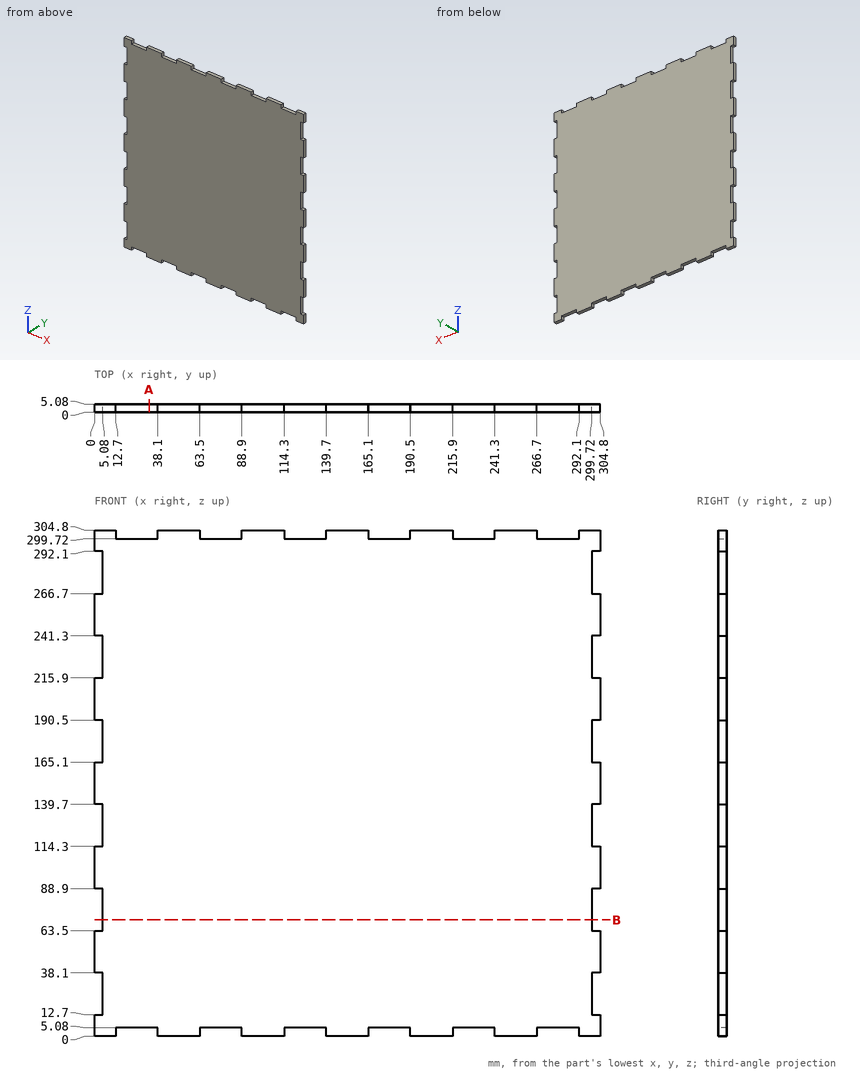
Print and shaded views of the part. All mm, measured from the part's lowest x, y and z. Round coordinates to 2 decimals unless told otherwise and drop trailing zeros. Write each loop counter-clockwise with the first axis right and the second up, starting at its lowest first coordinate (ties: lowest second). Pieces come first, ordered by that corner, then holes. Notation, with made-up numbers: (76.25, -17.5) -> (110.25, -17.5) arc R36 cw to (110.25, 16.5) -> close; hole circle Ø7 at (38.25, 53.5). An arc over 180 degrees is marked (long way). Answer in a Markdown table with one row per item. Add a question column.
Item 1: Saw through at A-A, the plane x = 33. Write the cut outline in (y, z).
Item 2: Drop a flat-ended pin along its axis: pin 1 Ø2.5 at (x, y) = (172.5, 2.5) entering from +Z. Give the stop position or say it passes through.
Item 3: Drill centre line: line 1 (X direction, y = 3.9, z = 186.5). Where is it in solid material? Low to high. Write a range as from..to.
Item 4: Saw through at B-B, the plane z = 70. Write the cut outline in (x, y).
Findings below:
| question | item | result |
|---|---|---|
| 1 | outline | (0, 5.08) -> (5.08, 5.08) -> (5.08, 299.72) -> (0, 299.72) -> close |
| 2 | pin 1 | stops at z = 299.72 |
| 3 | line 1 | x = 5.08..299.72 |
| 4 | outline | (5.08, 0) -> (299.72, 0) -> (299.72, 5.08) -> (5.08, 5.08) -> close |
